from build123d import *

# Parameters (mm, degrees)
F0_R     = 101.6
F1_DEPTH = 50.8
F2_R     = 38.1
F3_DEPTH = 50.8
F4_R     = 25.4
F5_DEPTH = 148.082
F6_R     = 12.7
F7_DEPTH = 95.758


with BuildPart() as f1:
    # F0 (on Front) → F1 (new body)
    with BuildSketch(Plane.XZ):
        Circle(F0_R)
    extrude(amount=F1_DEPTH)

    # F2 (on face) → F3 (join)
    with BuildSketch(Plane.XZ.offset(50.8)):
        Circle(F2_R)
    extrude(amount=F3_DEPTH)

    # F4 (on face) → F5 (cut)
    with BuildSketch(Plane.XZ.offset(101.6)):
        Circle(F4_R)
    extrude(amount=-F5_DEPTH, mode=Mode.SUBTRACT)

    # F6 (on face) → F7 (cut)
    with BuildSketch(Plane.XZ.offset(50.8)):
        with Locations((0, 76.2)):
            Circle(F6_R)
        with Locations((76.2, 0)):
            Circle(F6_R)
        with Locations((0, -76.2)):
            Circle(F6_R)
        with Locations((-76.2, 0)):
            Circle(F6_R)
    extrude(amount=-F7_DEPTH, mode=Mode.SUBTRACT)


solid = f1.part
Design review of the part built by this model. Coordinates are the model's own, in mm. A direction names the side the tool comes from. Coordinates: 2 decimals unless noted, no trailing zeros. Order: outer loops, then holes, each group sorted by start corner. A loop starts at its lowest first (then second) coordinate and runs counter-clockwise, first axis right, second up. Notation, with made-up numbers: (81.5, 54) -> (128.5, 54) arc R20 ccw to (128.5, 88) -> close; hole circle Ø7 at (88, 19). An arc over 180 degrees is marked (long way). Use one line per item in the form item = value. Start each with the question number.
(1) Insertion check: pin 1 (10 mm diameter, centred on x = 66, z = -37.5, fed in from -Y); pin 2 (1.5 mm diameter, centred on y = -53, z = 8, fed in from -X); pin 3 (4 mm diameter, centred on y = -30, z = 42, fed in from +X). Each pin has a flat end and moves straight along its axis. Give the tip position at first contact, or say it passes through.
(2) Add section A-A on x = 0. State the section outline as (y, z) points.
(3) Add section B-B on z = 4.5. State the section outline as (x, y) points.
(4) The part is to be moulded in two halves that separate along Z. For faces 3 (the cylindrical face through (12.114, -25.756, -72.385)), 4 (the flat face through (21, 0, -21)), 5 (the cylindrical face through (-22.025, -25.044, -99.184)), say which applies: +Z half, -Z half, draft (parallel to the pull), parting line (faces both ways), or undercut.
(5) Add section D-D on y = -14.5. State the section outline as (x, z) points.
(6) For faces 1 (the cylindrical face through (-30.235, -75.844, -23.183)), 2 (the cylindrical face through (-2.75, -25.76, 63.8)), list the 3-axis set-ups (+Z, -Z, +X, -X, +Y, -Y) from which the entire face can be reached by the end or side of a thin tool; tool diameter is ignored.
(7) For probe 1 along Z at (x, y) = (0, -37); probe 2 along X at (y, z) = (-11.5, -1.5); probe 3 along Z at (x, y) = (-8.5, -24), list the stretches that pass through material, from the lowest coordinate up.
(8) Add section C-C on x = -70.5. State the section outline as (y, z) points, plus the area to 3 significant figures.
Answer block:
q1.pin_1 = -50.8
q1.pin_2 = -37.4
q1.pin_3 = 93.39
q2.outline = (-101.6, -38.1) -> (-50.8, -38.1) -> (-50.8, -63.5) -> (0, -63.5) -> (0, -25.4) -> (-101.6, -25.4) -> close; (-101.6, 25.4) -> (0, 25.4) -> (0, 63.5) -> (-50.8, 63.5) -> (-50.8, 38.1) -> (-101.6, 38.1) -> close; (-50.8, -101.6) -> (0, -101.6) -> (0, -88.9) -> (-50.8, -88.9) -> close; (-50.8, 88.9) -> (0, 88.9) -> (0, 101.6) -> (-50.8, 101.6) -> close
q3.outline = (-101.5, -50.8) -> (-88.08, -50.8) -> (-88.08, 0) -> (-101.5, 0) -> close; (-64.32, -50.8) -> (-37.83, -50.8) -> (-37.83, -101.6) -> (-25, -101.6) -> (-25, 0) -> (-64.32, 0) -> close; (25, -101.6) -> (37.83, -101.6) -> (37.83, -50.8) -> (64.32, -50.8) -> (64.32, 0) -> (25, 0) -> close; (88.08, -50.8) -> (101.5, -50.8) -> (101.5, 0) -> (88.08, 0) -> close
q4.face_3 = undercut
q4.face_4 = draft
q4.face_5 = parting line
q5.outline = circle Ø203.2 at (0, 0); hole circle Ø25.4 at (-76.2, 0); hole circle Ø50.8 at (0, 0); hole circle Ø25.4 at (0, -76.2); hole circle Ø25.4 at (0, 76.2); hole circle Ø25.4 at (76.2, 0)
q6.face_1 = -Y
q6.face_2 = +Y, -Y
q7.probe_1 = -101.6 to -88.9, -63.5 to -25.4, 25.4 to 63.5, 88.9 to 101.6
q7.probe_2 = -101.59 to -88.81, -63.59 to -25.36, 25.36 to 63.59, 88.81 to 101.59
q7.probe_3 = -101.24 to -85.64, -66.76 to -23.94, 23.94 to 66.76, 85.64 to 101.24
q8.outline = (-50.8, -73.16) -> (0, -73.16) -> (0, -11.35) -> (-50.8, -11.35) -> close; (-50.8, 11.35) -> (0, 11.35) -> (0, 73.16) -> (-50.8, 73.16) -> close
q8.area = 6,280 mm²
